Work out the finished part from the listing and answer in its coordinate system (mm). A direction names the side the tool comes from. Give positions to 0.01 mm unless a question says otherwise; leave off trailing zeros. Order: outer loops, then holes, each group sorted by start corner. A loop starts at its lowest first (then second) coordinate and runs counter-clockwise, first axis right, second up. Notation, with made-up numbers: (-6, -29) -> (6, -29) arc R25 cw to (6, -8) -> close; hole circle Ø4 at (83, -35.75). An arc over 180 degrees is marked (long way). Answer as CSV lines item,"result". Start each with the question number.
1. For a pull along Z with two mould halves and no side action, classify faces 1 (the flat face through (0, 9.353, 3)), 2 (the cylindrical face through (-0.59, 4.46, 7.25)), 3 (the flat face through (2.4, -2.4, 0)) as released by +Z, released by -Z, zero draft, split by the parting line, or undercut.
2. For faces 4 (the flat face through (8.062, -4.742, 2.972)), 5 (the flat face through (-8.062, 4.742, 2.972)), 6 (the flat face through (0, -5, 7)), 7 (the flat face through (-8, -6, 1)), 8 (the flat face through (0, -9.353, 3)), determine the directions among +Z, -Z, +X, -X, +Y, -Y from which every point of the face is accessible in a straight line to the end or side of a thin tool.
3. Find the intervals of material crossed by L1, parallel to Y at x = 0, z = 3.5; L2, parallel to Z at x = -4, y = 7.25; L3, parallel to Y at x = -2.75, z = 7.75, in increasing order.
4. A cutting plane is placed at B-B (z = 2.25). Give the vertices of the cut face in (x, y), then the cut area to 3 significant figures.
5. A cutting plane is placed at D-D (y = 5.75). Give the vertices of the cut face in (x, z), then the cut area to 3 significant figures.
6. A cutting plane is placed at C-C (x = 6.5). Give the vertices of the cut face in (y, z).
7. Flat-ended cylindrical pins translate along their axes: pin 1 (4 mm diameter, centred on x = -1.5, z = 7.5, fed in from +Y); pin 2 (4.5 mm diameter, centred on x = -2, z = 3, fed in from -Y); pin 3 (4.5 mm diameter, centred on x = -2.5, z = 2.5, fed in from +Y). Find the tip coordinate at first contact, or state that the pin passes through.
8. A cutting plane is placed at A-A (x = 0). Give the vertices of the cut face in (y, z), then the cut area to 3 significant figures.
from build123d import *

# Parameters (mm, degrees)
F0_R      = 11.3
F1_DEPTH  = 1
F2_DEPTH  = 5
F3_R      = 7.25
F4_DEPTH  = 2
F5_R      = 4.5
F6_DEPTH  = 0.5
F7_R      = 5
F8_DEPTH  = 1.5
F9_R      = 3
F10_DEPTH = 13.7


with BuildPart() as f1:
    # F0 (on Top) → F1 (new body)
    with BuildSketch(Plane.XY):
        Circle(F0_R)
        Polygon((10.8, 0), (5.4, -9.353074), (-5.4, -9.353074), (-10.8, 0), (-5.4, 9.353074), (5.4, 9.353074), align=None, mode=Mode.SUBTRACT)
        Polygon((-5.4, -9.353074), (5.4, -9.353074), (10.8, 0), (5.4, 9.353074), (-5.4, 9.353074), (-10.8, 0), align=None)
    extrude(amount=F1_DEPTH)

    # F0 (on Top) → F2 (join)
    with BuildSketch(Plane.XY):
        Polygon((-5.4, -9.353074), (5.4, -9.353074), (10.8, 0), (5.4, 9.353074), (-5.4, 9.353074), (-10.8, 0), align=None)
    extrude(amount=F2_DEPTH)

    # F3 (on face) → F4 (join)
    with BuildSketch(Plane.XY.offset(5)):
        Circle(F3_R)
    extrude(amount=F4_DEPTH)

    # F5 (on face) → F6 (join)
    with BuildSketch(Plane.XY.offset(7)):
        Circle(F5_R)
    extrude(amount=F6_DEPTH)

    # F7 (on face) → F8 (join)
    with BuildSketch(Plane.XY.offset(7.5)):
        Circle(F7_R)
    extrude(amount=F8_DEPTH)

    # F9 (on face) → F10 (cut)
    with BuildSketch(Plane.XY.offset(9)):
        Circle(F9_R)
    extrude(amount=-F10_DEPTH, mode=Mode.SUBTRACT)


solid = f1.part
Answer sheet:
1,face 1,"zero draft"
1,face 2,"undercut"
1,face 3,"released by -Z"
2,face 4,"+Z, +X, -Y"
2,face 5,"+Z, -X, +Y"
2,face 6,"none"
2,face 7,"+Z"
2,face 8,"+Z, +X, -X, -Y"
3,L1,"y = -9.35 to -3, 3 to 9.35"
3,L2,"z = 0 to 5"
3,L3,"y = -4.18 to -1.2, 1.2 to 4.18"
4,outline,"(-10.8, 0) -> (-5.4, -9.35) -> (5.4, -9.35) -> (10.8, 0) -> (5.4, 9.35) -> (-5.4, 9.35) -> close; hole circle Ø6 at (0, 0)"
4,area,"275 mm^2"
5,outline,"(-9.73, 0) -> (9.73, 0) -> (9.73, 1) -> (7.48, 1) -> (7.48, 5) -> (4.42, 5) -> (4.42, 7) -> (-4.42, 7) -> (-4.42, 5) -> (-7.48, 5) -> (-7.48, 1) -> (-9.73, 1) -> close"
5,area,"97.0 mm^2"
6,outline,"(-9.24, 0) -> (9.24, 0) -> (9.24, 1) -> (7.45, 1) -> (7.45, 5) -> (3.21, 5) -> (3.21, 7) -> (-3.21, 7) -> (-3.21, 5) -> (-7.45, 5) -> (-7.45, 1) -> (-9.24, 1) -> close"
7,pin 1,"stops at y = 7.25"
7,pin 2,"stops at y = -11.26"
7,pin 3,"stops at y = 11.27"
8,outline,"(-11.3, 0) -> (-3, 0) -> (-3, 9) -> (-5, 9) -> (-5, 7.5) -> (-4.5, 7.5) -> (-4.5, 7) -> (-7.25, 7) -> (-7.25, 5) -> (-9.35, 5) -> (-9.35, 1) -> (-11.3, 1) -> close; (3, 0) -> (11.3, 0) -> (11.3, 1) -> (9.35, 1) -> (9.35, 5) -> (7.25, 5) -> (7.25, 7) -> (4.5, 7) -> (4.5, 7.5) -> (5, 7.5) -> (5, 9) -> (3, 9) -> close"
8,area,"91.9 mm^2"
